Build history of the part. All positions in model axes, mm. A direction names the side the tool comes from. Coordinates: 2 decimals unless noted, no trailing zeros. Loops run counter-clockwise (first coordinate to the right, second up) from the corner with the lowest first, then second, coordinate; pieces in that order, holes last.
(1) Slice it at A-A (z = 2). Give the cut face in (x, y).
(2) Wall check: L1, parallel to Y at x = 0, z = 4.5; L2, parallel to X at y = 0, z = 17; L3, parallel to Y at x = -4, z = 13.25. Give the ranges that are in metal, low to high.
(3) Two-plate mould, pull along Y, no slides. Class faces 3 (the face through (-6, -5, 0)), 4 (the face through (-7.593, 0.334, 5.916)), 5 (the face through (8.584, 2.703, 4.47)): pulls with the +Y half, pulls with the -Y half, needs draft (parallel to the pull), parting line crosses it, or undercut.
(4) Tool access for faces 1 (the face through (-15, 2, 24)), 2 (the face through (0, 5, 12)): list every direction of +Z, -Z, +X, -X, +Y, -Y with a clear straight run to the whole face (end or side of a thin tool).
(5) Flat gauge pins, fed straight in: P1, Ø6, axis at x = -7.5, z = 8.5, coming from the +Y side; P2, Ø2, axis at x = -8.5, z = 21, coming from the -Y side; P3, Ø4, axis at x = -3.5, z = 10.5, coming from the +Y side. Where does each tip first touch, or does it go through?
(6) Slice it at B-B (z = 16.25). Give the cut face in (x, y).
from build123d import *

# Parameters (mm, degrees)
F0_R     = 9
F0_R_2   = 7.6
F3_DEPTH = 12
F5_R     = 10


# Not quite as in the source:
# - a feature names something its author has since deleted; it is built from what else it names


with BuildPart() as f3:
    # F0 (on Top) → F3 (new body)
    with BuildSketch(Plane.XY):
        Circle(F0_R)
        Circle(F0_R_2, mode=Mode.SUBTRACT)
    extrude(amount=F3_DEPTH)

    # F1 (on Front) → F4 (revolve)
    with BuildSketch(Plane.XZ):
        Polygon((14.9, 24), (4.5, 12), (9, 12), (16.7, 24), align=None)
    revolve(axis=Axis((0, 0, -6.017471198), (0, 0, -1)))

    # F5
    f5_edges = [f3.edges().sort_by_distance(p)[0] for p in [
        (-9, 0, 12),
    ]]
    fillet(f5_edges, radius=F5_R)


solid = f3.part
Response values:
1. outline: circle Ø18 at (0, 0); hole circle Ø15.2 at (0, 0)
2. L1: y = -9 to -7.6, 7.6 to 9
2. L2: x = -12.21 to -8.83, 8.83 to 12.21
2. L3: y = -9.07 to -3.9, 3.9 to 9.07
3. face 3: needs draft
3. face 4: undercut
3. face 5: parting line crosses it
4. face 1: +Z, +X, -X, +Y, -Y
4. face 2: -Z
5. P1: stops at y = 7.79
5. P2: stops at y = -13.09
5. P3: stops at y = 9.19
6. outline: circle Ø23.45 at (0, 0); hole circle Ø16.37 at (0, 0)
